from build123d import *

# Parameters (mm, degrees)
SKETCH1_W                      = 94
SKETCH1_H                      = 130
BOSS_EXTRUDE1_DEPTH            = 35
SKETCH2_W                      = 90.5
SKETCH2_H                      = 126.5
BOSS_EXTRUDE2_DEPTH            = 2.5
CUT_EXTRUDE1_DEPTH             = 38.5
SKETCH4_W                      = 5
SKETCH4_H                      = 18
CUT_EXTRUDE2_DEPTH             = 5
SKETCH9_W                      = 5
SKETCH9_H                      = 18
CUT_EXTRUDE6_DEPTH             = 5
SKETCH11_W                     = 5
SKETCH11_H                     = 5
CUT_EXTRUDE8_DEPTH             = 18
SKETCH12_W                     = 5
SKETCH12_H                     = 18
CUT_EXTRUDE9_DEPTH             = 5
F_5_5_5_5_DIAMETER_HOLE1_D     = 5.5
F_5_5_5_5_DIAMETER_HOLE1_DEPTH = 5
FILLET1_R                      = 2
CUT_EXTRUDE10_DEPTH            = 2.5
SKETCH17_W                     = 40
SKETCH17_H                     = 6
BOSS_EXTRUDE3_DEPTH            = 8
SKETCH18_W                     = 40
SKETCH18_H                     = 6
BOSS_EXTRUDE4_DEPTH            = 8
SKETCH23_R                     = 1.5
CUT_EXTRUDE11_DEPTH            = 4.4


with BuildPart() as part:
    # Sketch1 → Boss-Extrude1 (new body)
    with BuildSketch(Plane.XZ):
        with Locations((47, -65)):
            Rectangle(SKETCH1_W, SKETCH1_H)
    extrude(amount=-BOSS_EXTRUDE1_DEPTH)

    # Sketch2 → Boss-Extrude2 (add)
    with BuildSketch(Plane(origin=(0, 35, 0), x_dir=(-1, 0, 0), z_dir=(0, 1, 0))):
        with Locations((-47, -65)):
            Rectangle(SKETCH2_W, SKETCH2_H)
    extrude(amount=BOSS_EXTRUDE2_DEPTH)

    # Sketch3 → Cut-Extrude1 (cut, through all)
    with BuildSketch(Plane(origin=(0, 37.5, 0), x_dir=(-1, 0, 0), z_dir=(0, 1, 0))):
        Polygon((-83, -120), (-79, -120), (-79, -125), (-15, -125), (-15, -120), (-5, -120), (-5, -10), (-15, -10), (-15, -5), (-79, -5), (-79, -10), (-89, -10), (-89, -96), (-89, -120), align=None)
    extrude(amount=-CUT_EXTRUDE1_DEPTH, mode=Mode.SUBTRACT)

    # Sketch4 → Cut-Extrude2 (cut)
    with BuildSketch(Plane(origin=(0, 0, -10), x_dir=(-1, 0, 0), z_dir=(0, 0, -1))):
        with Locations((-12.5, 9)):
            Rectangle(SKETCH4_W, SKETCH4_H)
    extrude(amount=-CUT_EXTRUDE2_DEPTH, mode=Mode.SUBTRACT)

    # Sketch9 → Cut-Extrude6 (cut)
    with BuildSketch(Plane(origin=(0, 0, -10), x_dir=(-1, 0, 0), z_dir=(0, 0, -1))):
        with Locations((-81.5, 9)):
            Rectangle(SKETCH9_W, SKETCH9_H)
    extrude(amount=-CUT_EXTRUDE6_DEPTH, mode=Mode.SUBTRACT)

    # Sketch11 → Cut-Extrude8 (cut)
    with BuildSketch(Plane.XZ):
        with Locations((12.5, -122.5)):
            Rectangle(SKETCH11_W, SKETCH11_H)
    extrude(amount=-CUT_EXTRUDE8_DEPTH, mode=Mode.SUBTRACT)

    # Sketch12 → Cut-Extrude9 (cut)
    with BuildSketch(Plane.XY.offset(-120)):
        with Locations((81.5, 9)):
            Rectangle(SKETCH12_W, SKETCH12_H)
    extrude(amount=-CUT_EXTRUDE9_DEPTH, mode=Mode.SUBTRACT)

    # Ø5.5 (5.5) Diameter Hole1
    with Locations(Plane(origin=(0, 0, -5), x_dir=(-1, 0, 0), z_dir=(0, 0, -1))):
        with Locations((-22, 10)):
            Hole(F_5_5_5_5_DIAMETER_HOLE1_D / 2, depth=F_5_5_5_5_DIAMETER_HOLE1_DEPTH)

    # Fillet1
    fillet1_edges = [part.edges().sort_by_distance(p)[0] for p in [
        (94, 17.5, -130),
        (0, 17.5, -130),
        (0, 17.5, 0),
        (94, 17.5, 0),
    ]]
    fillet(fillet1_edges, radius=FILLET1_R)

    # Sketch16 → Cut-Extrude10 (cut)
    with BuildSketch(Plane.XZ):
        with BuildLine():
            Line((0, -2), (0, -128))
            ThreePointArc((0, -128), (0.585786438, -129.414213562), (2, -130))
            Line((2, -130), (92, -130))
            ThreePointArc((92, -130), (93.414213562, -129.414213562), (94, -128))
            Line((94, -128), (94, -2))
            ThreePointArc((94, -2), (93.414213562, -0.585786438), (92, 0))
            Line((92, 0), (2, 0))
            ThreePointArc((2, 0), (0.585786438, -0.585786438), (0, -2))
        make_face()
        with BuildLine():
            Line((1.5, -2), (1.5, -128))
            ThreePointArc((1.5, -128), (1.646446609, -128.353553391), (2, -128.5))
            Line((2, -128.5), (92, -128.5))
            ThreePointArc((92, -128.5), (92.353553391, -128.353553391), (92.5, -128))
            Line((92.5, -128), (92.5, -2))
            ThreePointArc((92.5, -2), (92.353553391, -1.646446609), (92, -1.5))
            Line((92, -1.5), (2, -1.5))
            ThreePointArc((2, -1.5), (1.646446609, -1.646446609), (1.5, -2))
        make_face(mode=Mode.SUBTRACT)
    extrude(amount=-CUT_EXTRUDE10_DEPTH, mode=Mode.SUBTRACT)

    # Sketch17 → Boss-Extrude3 (add)
    with BuildSketch(Plane(origin=(5, 0, 0), x_dir=(0, 0, -1), z_dir=(1, 0, 0))):
        with Locations((100, 32.9)):
            Rectangle(SKETCH17_W, SKETCH17_H)
    extrude(amount=BOSS_EXTRUDE3_DEPTH)

    # Sketch18 → Boss-Extrude4 (add)
    with BuildSketch(Plane.ZY.offset(-89)):
        with Locations((-100, 32.9)):
            Rectangle(SKETCH18_W, SKETCH18_H)
    extrude(amount=BOSS_EXTRUDE4_DEPTH)

    # Sketch23 → Cut-Extrude11 (cut)
    with BuildSketch(Plane(origin=(0, 35.9, 0), x_dir=(1, 0, 0), z_dir=(0, 1, 0))):
        with Locations((9.61875, 115.175)):
            Circle(SKETCH23_R)
        with Locations((9.61875, 85.0125)):
            Circle(SKETCH23_R)
        with Locations((84.23125, 115.175)):
            Circle(SKETCH23_R)
        with Locations((84.23125, 85.0125)):
            Circle(SKETCH23_R)
    extrude(amount=-CUT_EXTRUDE11_DEPTH, mode=Mode.SUBTRACT)


solid = part.part
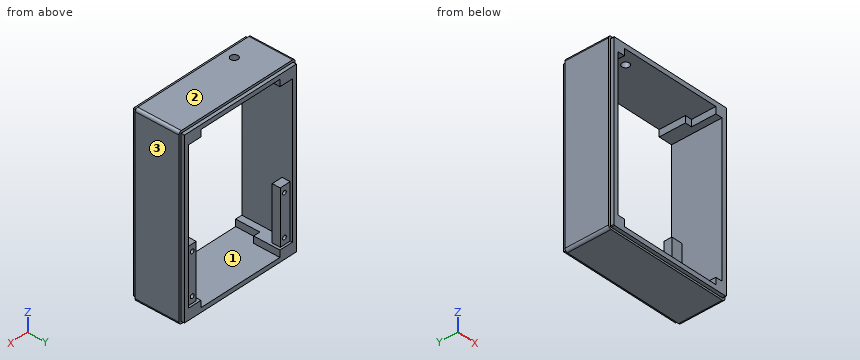
The listing builds one solid part. Answer for the finished solid, in the listing's coordinates (mm). Face numbers are marked on the shaded views. Coordinates: 2 decimals unless noted, no trailing zeros. Write each loop counter-clockwise with the first axis right and the second up, starting at its lowest first coordinate (ties: lowest second). Pieces come first, ordered by that corner, then holes. Notation, with made-up numbers: M 73.5,-32 L 129.5,-32 A10 cw 129.5,-17 Z; hole C 46,-17.5 d11. An arc over 180 degrees is marked long. Use one line per item in the form item = value.
Item 1: Find section D-D, the plane y = 10. Give the vertices of the cut face in (x, z).
Model answer:
outline = M 0,-128 A2 ccw 2,-130 L 92,-130 A2 ccw 94,-128 L 94,-2 A2 ccw 92,0 L 24.75,0 L 24.75,-5 L 84,-5 L 84,-10 L 89,-10 L 89,-120 L 84,-120 L 84,-125 L 10,-125 L 10,-120 L 5,-120 L 5,-10 L 10,-10 L 10,-5 L 19.25,-5 L 19.25,0 L 2,0 A2 ccw 0,-2 Z
Item 2: Find section A-A, the plane x = 22. Give the vertices of the cut face in (y, z).
Model answer:
outline = M 0,-128.5 L 2.5,-128.5 L 2.5,-130 L 35,-130 L 35,-128.25 L 37.5,-128.25 L 37.5,-125 L 0,-125 Z; M 0,-5 L 7.25,-5 L 7.25,0 L 2.5,0 L 2.5,-1.5 L 0,-1.5 Z; M 12.75,-5 L 37.5,-5 L 37.5,-1.75 L 35,-1.75 L 35,0 L 12.75,0 Z
Item 3: The mould has two halves that part along X. Classify the marked faces 1, 2 and 3: released by +X, released by -X, zero draft, split by the parting line, or undercut.
Model answer:
face_1 = undercut
face_2 = zero draft
face_3 = released by +X
Item 4: Given P1, Ø3, axis at x = 53.5, y = 37, coming from the -Z side; P2, Ø2.5, axis at x = 82.5, z = -7, coming from the -Y side; P3, Ø3.5, axis at x = 10, z = -115, coming from the +Y side; P4, Ø6, axis at x = 84, z = -57, coming from the -Y side, each flat-ended and moving along its own axis, determine where each tip first touches the part or whether it passes through.
Model answer:
P1 = -128.25
P2 = 18
P3 = 35.9
P4 = through
Item 5: Find section C-C, the plane z = -34. Give the vertices of the cut face in (x, y).
Model answer:
outline = M 0,2.5 L 1.5,2.5 L 1.5,0 L 5,0 L 5,37.5 L 1.75,37.5 L 1.75,35 L 0,35 Z; M 89,0 L 92.5,0 L 92.5,2.5 L 94,2.5 L 94,35 L 92.25,35 L 92.25,37.5 L 89,37.5 Z
Item 6: Find section B-B, the plane y = 27.5. Give the vertices of the cut face in (x, z), plus the area to 3 significant figures.
Model answer:
outline = M 0,-128 A2 ccw 2,-130 L 92,-130 A2 ccw 94,-128 L 94,-2 A2 ccw 92,0 L 2,0 A2 ccw 0,-2 Z; hole M 5,-120 L 15,-120 L 15,-125 L 79,-125 L 79,-120 L 89,-120 L 89,-10 L 79,-10 L 79,-5 L 15,-5 L 15,-10 L 5,-10 Z
area = 2,340 mm2
Item 7: Find the intervals of material crossed by probe 1 along X at (y, z) = (33.5, -12); probe 2 along X at (y, z) = (30, -119.5); probe 3 along Z at (x, y) = (45.5, 28), in increasing order.
Model answer:
probe_1 = 0 to 5, 89 to 94
probe_2 = 0 to 13, 81 to 94
probe_3 = -130 to -125, -5 to 0
